```python
from build123d import *

# Parameters (mm, degrees)
F0_W      = 65
F0_H      = 30
F2_DEPTH  = 2
F3_R      = 3
F4_R      = 1.375
F5_DEPTH  = 2
F8_W      = 10.42
F8_H      = 4.8704799486
F8_H_2    = 0.4562667193
F9_DEPTH  = 2.42
F8_W_2    = 6.85
F10_DEPTH = 1.8
F8_W_3    = 14.6107960276
F8_H_3    = 11
F8_W_4    = 0.3892039724
F11_DEPTH = 1
F8_W_5    = 4
F8_H_4    = 17
F12_DEPTH = 1
F13_W     = 5
F13_H     = 4.9290289432
F15_DEPTH = 8


with BuildPart() as f2:
    # F0 (on Top) → F2 (new body)
    with BuildSketch(Plane.XY):
        with Locations((-7.9789588384, 18.2161135599)):
            Rectangle(F0_W, F0_H)
    extrude(amount=F2_DEPTH)

    # F3
    f3_edges = [f2.edges().sort_by_distance(p)[0] for p in [
        (-40.478959, 33.216114, 1),
        (-40.478959, 3.216114, 1),
        (24.521041, 3.216114, 1),
        (24.521041, 33.216114, 1),
    ]]
    fillet(f3_edges, radius=F3_R)

    # F4 (on face) → F5 (cut)
    with BuildSketch(Plane.XY.offset(2)):
        with Locations((21.0210420191, 29.7161135823)):
            Circle(F4_R)
        with Locations((-36.9789588384, 6.7161135599)):
            Circle(F4_R)
        with Locations((-36.9789588384, 29.7161135823)):
            Circle(F4_R)
        with Locations((21.0210411616, 6.7161135599)):
            Circle(F4_R)
    extrude(amount=-F5_DEPTH, mode=Mode.SUBTRACT)

    # F8 (on face) → F9 (join)
    with BuildSketch(Plane.XY.offset(2)):
        with Locations((-28.0789588384, 5.6513535342)):
            Rectangle(F8_W, F8_H)
        with Locations((-28.0789588384, 2.9879802003)):
            Rectangle(F8_W, F8_H_2)
    extrude(amount=F9_DEPTH)

    # F8 (on face) → F10 (join)
    with BuildSketch(Plane.XY.offset(2)):
        with Locations((0.9210411616, 5.6513535342)):
            Rectangle(F8_W_2, F8_H)
        with Locations((13.5210411616, 5.6513535342)):
            Rectangle(F8_W_2, F8_H)
        with Locations((0.9210411616, 2.9879802003)):
            Rectangle(F8_W_2, F8_H_2)
        with Locations((13.5210411616, 2.9879802003)):
            Rectangle(F8_W_2, F8_H_2)
    extrude(amount=F10_DEPTH)

    # F8 (on face) → F11 (join)
    with BuildSketch(Plane.XY.offset(2)):
        with Locations((-33.1735608246, 20.1161135599)):
            Rectangle(F8_W_3, F8_H_3)
        with Locations((-40.6735608246, 20.1161135599)):
            Rectangle(F8_W_4, F8_H_3)
    extrude(amount=F11_DEPTH)

    # F8 (on face) → F12 (join)
    with BuildSketch(Plane.XY.offset(2)):
        with Locations((22.5210411616, 18.2120301798)):
            Rectangle(F8_W_5, F8_H_4)
    extrude(amount=F12_DEPTH)

    # F13 (on face) → F15 (join)
    with BuildSketch(Plane.XY.offset(2)):
        Polygon((12.5210411616, 26.7161135823), (17.5210411616, 26.7161135823), (17.5210411616, 32.7161135823), (-33.4789588384, 32.7161135823), (-33.4789588384, 26.7161135823), align=None)
        with Locations((15.0210411616, 24.2515991107)):
            Rectangle(F13_W, F13_H)
    extrude(amount=F15_DEPTH)


solid = f2.part
```
For this review, take the finished solid that the model builds, in its own axes (mm). A direction names the side the tool comes from. Coordinates: 2 decimals unless noted, no trailing zeros. Loops run counter-clockwise (first coordinate to the right, second up) from the corner with the lowest first, then second, coordinate; pieces in that order, holes last. Notation, with made-up numbers: (15.5, 9.25) -> (30.5, 9.25) arc R19 cw to (30.5, 21.25) -> close; hole circle Ø4 at (4.25, -12). An arc over 180 degrees is marked (long way). Return JSON: item names as keys, results as strings. Group by question number.
(1) Tool access review of faces 4 (the flat face through (-33, 20, 3)), 5 (the flat face through (10.096, 5, 3)), 6 (the flat face through (-8, 32.716, 6)): name each direction out of +Z, -Z, +X, -X, +Y, -Y from which nothing blocks a thin tool from reaching the whole face with its end or side.
(2) To check wall thickness, follow L1, parallel to Z at x = -18, y = 19; L2, parallel to Y at x = -12.5, z = 6; L3, parallel to Y at x = 15.5, z = 8.5. State the ranges of each line that lie inside material, in increasing order.
(3) Consider section C-C, the plane z = 6.75. Give the boundary of the cut face in (x, y), plus the area to 3 significant figures.
(4) Consider section A-A, the plane x = 3. Give the boundary of the cut face in (y, z).
(5) Consider section D-D, the plane x = -28.5. Give the boundary of the cut face in (y, z).
(6) Mouldability with a two-part tool opening along Y and no side actions: class faces 1 (the flat face through (1, 2.76, 3)), 2 (the flat face through (22, 18, 3)), 3 (the flat face through (13, 8.087, 3)) as pulls with the +Y half, pulls with the -Y half, needs draft (parallel to the pull), parting line crosses it, or undercut.
(7) For pin 1 Ø3.5 at (x, y) = (-34, 22) entering from +Z; pin 2 Ø1 at (x, z) = (-4.5, 1) entering from -Y; pin 3 Ø2 at (x, z) = (0, 3.5) entering from +Y, all flat-tipped, find the tip position at first contact; note any pin that passes through.
(8) Consider section B-B, the plane y = 21. Give the boundary of the cut face in (x, z).
Results below:
{
 "1": {"face 4": "+Z, -X", "face 5": "+Z, -Y", "face 6": "+Z, +X, -X, +Y"},
 "2": {"L1": "z = 0 to 2", "L2": "y = 26.72 to 32.72", "L3": "y = 21.79 to 32.72"},
 "3": {"outline": "(-33.48, 26.72) -> (12.52, 26.72) -> (12.52, 21.79) -> (17.52, 21.79) -> (17.52, 32.72) -> (-33.48, 32.72) -> close", "area": "331 mm2"},
 "4": {"outline": "(2.76, 2) -> (3.22, 2) -> (3.22, 0) -> (33.22, 0) -> (33.22, 2) -> (32.72, 2) -> (32.72, 10) -> (26.72, 10) -> (26.72, 2) -> (8.09, 2) -> (8.09, 3.8) -> (2.76, 3.8) -> close"},
 "5": {"outline": "(2.76, 2) -> (3.22, 2) -> (3.22, 0) -> (33.22, 0) -> (33.22, 2) -> (32.72, 2) -> (32.72, 10) -> (26.72, 10) -> (26.72, 2) -> (25.62, 2) -> (25.62, 3) -> (14.62, 3) -> (14.62, 2) -> (8.09, 2) -> (8.09, 4.42) -> (2.76, 4.42) -> close"},
 "6": {"face 1": "pulls with the -Y half", "face 2": "needs draft", "face 3": "undercut"},
 "7": {"pin 1": "stops at z = 3", "pin 2": "stops at y = 3.22", "pin 3": "stops at y = 32.72"},
 "8": {"outline": "(-40.87, 2) -> (-40.48, 2) -> (-40.48, 0) -> (24.52, 0) -> (24.52, 3) -> (20.52, 3) -> (20.52, 2) -> (-25.87, 2) -> (-25.87, 3) -> (-40.87, 3) -> close"}
}
